Work out the finished part from the listing and answer in its coordinate system (mm). A direction names the side the tool comes from. Round coordinates to 2 decimals unless told otherwise and drop trailing zeros. Write each loop counter-clockwise with the first axis right and the second up, starting at its lowest first coordinate (ties: lowest second). Pieces come first, ordered by that corner, then holes.
Autodesk Inventor part; units mm, degrees
ref_plane "YZ Plane" through (0, 0, 0) normal (1, 0, 0) x (0, 1, 0)
ref_plane "XZ Plane" through (0, 0, 0) normal (0, 1, 0) x (-1, 0, 0)
ref_plane "XY Plane" through (0, 0, 0) normal (0, 0, 1) x (1, 0, 0)
sketch "Esboço1" plane through (0, 0, 0) normal (0, 0, 1) x (1, 0, 0)
  line L0 (-195, -120) -> (-195, 120)
  line L1 (-195, 120) -> (195, 120)
  line L2 (195, 120) -> (195, -120)
  line L3 (195, -120) -> (-195, -120)
  line L4 (0, 168.2) -> (0, -169.2) construction
  line L5 (-273, 0) -> (273, 0) construction
  line L6 (175, 100) -> (175, -80)
  line L7 (175, -80) -> (-175, -80)
  line L8 (-175, -80) -> (-175, 100)
  line L9 (-175, 100) -> (175, 100)
  line L10 (185, 110) -> (185, -90) construction
  line L11 (185, -90) -> (-185, -90) construction
  line L12 (-185, -90) -> (-185, 110) construction
  line L13 (-185, 110) -> (185, 110) construction
  line L14 (185.25, 110.25) -> (185.25, -90.25)
  line L15 (185.25, -90.25) -> (-185.25, -90.25)
  line L16 (-185.25, -90.25) -> (-185.25, 110.25)
  line L17 (-185.25, 110.25) -> (185.25, 110.25)
  circle A0 centre (183.25, 108.25) radius 3
  circle A1 centre (-183.25, 108.25) radius 3
  line L18 (175, 10) -> (-175, 10) construction
  circle A2 centre (183.25, -88.25) radius 3
  circle A3 centre (-183.25, -88.25) radius 3
  line L19 (180, 105) -> (180, -85) construction
  line L20 (180, -85) -> (-180, -85) construction
  line L21 (-180, -85) -> (-180, 105) construction
  line L22 (-180, 105) -> (180, 105) construction
  line L23 (159.5, -104) -> (159.5, -120)
  line L24 (159.5, -120) -> (120.5, -120)
  line L25 (120.5, -120) -> (120.5, -104)
  line L26 (120.5, -104) -> (159.5, -104)
  line L27 (140, -104) -> (140, -120) construction
  line L28 (159.5, -112) -> (120.5, -112) construction
  circle A4 centre (123.5, -104) radius 3
  line L29 (-159.5, -104) -> (-159.5, -120)
  line L30 (-159.5, -120) -> (-120.5, -120)
  line L31 (-120.5, -120) -> (-120.5, -104)
  line L32 (-120.5, -104) -> (-159.5, -104)
  line L33 (-140, -105) -> (-140, -121) construction
  line L34 (-159.5, -112) -> (-120.5, -112) construction
  circle A5 centre (-156.5, -104) radius 3
  circle A6 centre (-123.5, -104) radius 3
  circle A7 centre (156.5, -104) radius 3
  point P0 (0, 0)
  point P1 (0, -85)
  point P2 (-180, 10)
  point P3 (180, 10)
  point P4 (0, 105)
  point P5 (151.5, -112)
  point P6 (128.5, -112)
  point P7 (-151.5, -112)
  point P8 (-128.5, -112)
  point P9 (-181.0139, 110.25)
  point P10 (-185.25, 106.0139)
  point P11 (-185.25, -86.0139)
  point P12 (-181.0139, -90.25)
  point P13 (181.0139, -90.25)
  point P14 (185.25, -86.0139)
  point P15 (185.25, 106.0139)
  point P16 (181.0139, 110.25)
  point P17 (159.5, -120)
  point P18 (126.5, -104)
  point P19 (-153.5, -104)
  point P20 (-159.5, -120)
  point P21 (-126.5, -104)
  point P22 (-90, 105)
  point P23 (90, 105)
  point P24 (-90, -85)
  point P25 (90, -85)
  point P26 (106.5, -104)
  point P27 (153.5, -104)
  dimension "d112" = 10
  dimension "d113" = 0.25
  dimension "d114" = 6
  dimension "d115" = 2
  dimension "d116" = 2
  dimension "d117" = 5
  dimension "d123" = 16
  dimension "d124" = 8
  dimension "d125" = 39
  dimension "d126" = 280
  dimension "d127" = 240
  dimension "d128" = 390
  dimension "d129" = 20
  dimension "d130" = 200
  dimension "d131" = 350
  dimension "d132" = 10
  dimension "d133" = 0.25
  dimension "d134" = 5
  dimension "d163" = 90
  dimension "d164" = 90
  dimension "d165" = 23
  dimension "d166" = 370
extrude "Extrusão1" add sketch "Esboço1" against normal blind 10 contours L0 L1 L2 L3 L23 A7 L26 A4 L25 L31 A6 L32 A5 L29 | L29 A5 L32 A6 L31 L3 | A5 L32 | L32 A5 | L25 A4 L26 A7 L23 L3 | A6 L32 | L32 A6 | A4 L26 | L26 A4 | A7 L26 | L26 A7 | L6 L7 L8 L9 | L17 A0 L14 | L14 A0 L17 | L14 A2 L15 A3 L16 A1 L17 A0 | A2 L15 L14 | L14 L15 A2 | A1 L16 L17 | L17 L16 A1 | A3 L16 L15 | L15 L16 A3
extrude "Extrusion13" cut sketch "Esboço1" against normal blind 0.2 contours L6 L7 L8 L9 | L17 A0 L14 | L14 A0 L17 | L14 A2 L15 A3 L16 A1 L17 A0 | A2 L15 L14 | L14 L15 A2 | A1 L16 L17 | L17 L16 A1 | A3 L16 L15 | L15 L16 A3
extrude "Extrusion14" cut sketch "Esboço1" against normal blind 1.3 contours L29 A5 L32 A6 L31 L3 | A5 L32 | L32 A5 | L25 A4 L26 A7 L23 L3 | A6 L32 | L32 A6 | A4 L26 | L26 A4 | A7 L26 | L26 A7
extrude "Extrusion15" cut sketch "Esboço1" against normal through all contours L6 L7 L8 L9
hole "Hole4" at (-151.5, -112, 0) at (-128.5, -112, 0) at (128.5, -112, 0) at (151.5, -112, 0) direction (0, 0, -1) diameter 2.459 end through all
hole "Hole5" at (0, -85, 0) at (-180, -85, 0) at (-180, 10, 0) at (180, -85, 0) at (180, 10, 0) at (-180, 105, 0) at (0, 105, 0) at (180, 105, 0) at (90, -85, 0) at (90, 105, 0) at (-90, 105, 0) at (-90, -85, 0) direction (0, 0, -1) diameter 3.242 end through all
fillet "Fillet2" radius 2 20 edges at (-185.25, -86.0139, -0.1) (-181.0139, -90.25, -0.1) (-185.25, 106.0139, -0.1) (-181.0139, 110.25, -0.1) (181.0139, 110.25, -0.1) (185.25, 106.0139, -0.1) (181.0139, -90.25, -0.1) (185.25, -86.0139, -0.1) (-153.5, -104, -0.65) (-126.5, -104, -0.65) (195, -120, -5) (-195, -120, -5) (-195, 120, -5) (195, 120, -5) (153.5, -104, -0.65) (159.5, -120, -0.65) (120.5, -120, -0.65) (-159.5, -120, -0.65) (-120.5, -120, -0.65) (126.5, -104, -0.65)
fillet "Fillet2" radius 5 4 edges at (-175, 100, -5.1) (-175, -80, -5.1) (175, -80, -5.1) (175, 100, -5.1)
chamfer "Chamfer2" distance 1 angle 45 4 edges at (-151.5, -110.7705, -1.3) (-128.5, -110.7705, -1.3) (128.5, -110.7705, -1.3) (151.5, -110.7705, -1.3)
equation "\"d115\" = 0.333333 * d114"
equation "\"d116\" = d115"
properties part number "GRJ-04-105" material "Fenolite OR"
Q1. Given pin 1 (3 mm diameter, centred on x = -180, y = -85, fed in from +Z); pin 2 (15 mm diameter, centred on x = -147.5, y = -114, fed in from +Z); pin 3 (4 mm diameter, centred on x = -151.5, y = -112, fed in from +Z); pin 4 (4 mm diameter, centred on x = 128.5, y = -112, fed in from -Z), each flat-ended and moving along its own axis, determine where each tip first touches the part or whether it passes through.
Q2. A tool of negligible diameter and unlimited length cuts with its end or side. For faces 5 (the face through (140, -110, -1.3)), 6 (the face through (175, 11, -5)), from which of +Z, -Z, +X, -X, +Y, -Y can it reach the whole face along a straight path? Write none if from no direction.
Q3. Find section C-C (z = -5). Count the separate pieces of the cut face and the enclosed holes in it, plus the area to 3 significant figures.
Q4. Find section B-B (y = -44.5). Determine the outline of the cut face in (x, z).
Q5. Find the intervals of material crossed by L1, parallel to X at y = -85, z = -2.5; L2, parallel to Y at x = -90, z = -6; L3, parallel to Y at x = 33.5, z = -2, in increasing order.
Q6. Find section A-A (x = 47). Determine the outline of the cut face in (y, z).
Q7. The mould has two halves that part along Y. Classify faces 1 (the face through (3, -120, -5)), 2 (the face through (2, -80, -5)), 3 (the face through (-3, 120, -5)), 4 (the face through (-195, -2, -5)): +Y half, -Y half, draft (parallel to the pull), parting line (faces both ways), or undercut.
Report:
1. pin 1: passes through
1. pin 2: stops at z = -1.3
1. pin 3: stops at z = -1.53
1. pin 4: stops at z = -10
2. face 5: +Z, -Y
2. face 6: +Z, -Z
3. separate pieces: 1
3. enclosed holes: 17
3. area: 30,500 mm2
4. outline: (-195, -10) - (-175, -10) - (-175, -0.2) - (-185.25, -0.2) - (-185.25, 0) - (-195, 0) - close; (175, -10) - (195, -10) - (195, 0) - (185.25, 0) - (185.25, -0.2) - (175, -0.2) - close
5. L1: x = -195 to -181.62, -178.38 to -91.62, -88.38 to -1.62, 1.62 to 88.38, 91.62 to 178.38, 181.62 to 195
5. L2: y = -120 to -86.62, -83.38 to -80, 100 to 103.38, 106.62 to 120
5. L3: y = -120 to -80, 100 to 120
6. outline: (-120, -10) - (-80, -10) - (-80, -0.2) - (-90.25, -0.2) - (-90.25, 0) - (-120, 0) - close; (100, -10) - (120, -10) - (120, 0) - (110.25, 0) - (110.25, -0.2) - (100, -0.2) - close
7. face 1: -Y half
7. face 2: undercut
7. face 3: +Y half
7. face 4: draft
